Check sheet for the modelled part. Datum: model origin and axes. Units: mm. Face numbers are marked on the shaded views. A direction names the side the tool comes from. Coordinates: 2 decimals unless noted, no trailing zeros. Write each loop counter-clockwise with the first axis right and the second up, starting at its lowest first coordinate (ties: lowest second). Pieces come first, ordered by that corner, then holes. Notation, with made-up numbers: (76, 49) - (109, 49) arc R15 cw to (109, 55) - close; hole circle Ø4 at (65.5, -35.75). An arc over 180 degrees is marked (long way). Write each question's results on one line, items separated by ' | '.
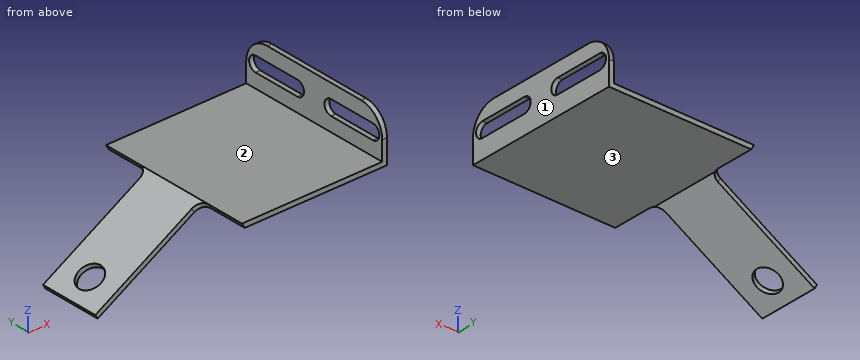
Autodesk Inventor part; units mm, degrees
ref_plane "YZ Plane" through (0, 0, 0) normal (1, 0, 0) x (0, 1, 0)
ref_plane "XZ Plane" through (0, 0, 0) normal (0, 1, 0) x (-1, 0, 0)
ref_plane "XY Plane" through (0, 0, 0) normal (0, 0, 1) x (1, 0, 0)
sketch "Skizze1" plane through (0, 0, 0) normal (0, 1, 0) x (-1, 0, 0)
  line L0 (0, 0) -> (0, -2)
  line L1 (0, -2) -> (60, -2)
  line L2 (60, -2) -> (103.3013, -27)
  line L3 (103.3013, -27) -> (104.3013, -25.2679)
  line L4 (0, 0) -> (60.5359, 0)
  line L5 (104.3013, -25.2679) -> (60.5359, 0)
  dimension "d0" = 2
  dimension "d1" = 60
  dimension "d2" = 50
  dimension "d3" = 150
  dimension "d4" = 2
  dimension "d42" = 0
extrude "Extrusion1" add sketch "Skizze1" along normal blind 65
sketch "Skizze2" plane through (-60.5359, 0, 0) normal (0, 0, 1) x (1, 0, 0)
  line L0 (60.5359, 0) -> (0.5359, 0)
  line L1 (60.5359, 0) -> (58.5359, 0)
  line L2 (58.5359, 0) -> (58.5359, 65)
  line L3 (58.5359, 65) -> (60.5359, 65)
  line L4 (60.5359, 65) -> (60.5359, 0)
  point P0 (58.5359, 0)
  dimension "d8" = 2
  dimension "d9" = 65
extrude "Extrusion2" add sketch "Skizze2" along normal blind 18
sketch "Skizze3" plane through (-2, 0, 0) normal (-1, 0, 0) x (0, 0, 1)
  line L0 (0, 0) -> (18, 0)
  line L1 (18, 65) -> (18, 0)
  line L2 (9, 24.5) -> (9, 4.5) construction
  line L3 (5.9, 24.5) -> (5.9, 4.5)
  line L4 (12.1, 4.5) -> (12.1, 24.5)
  arc A0 (12.1, 24.5) -> (5.9, 24.5) centre (9, 24.5) ccw
  arc A1 (5.9, 4.5) -> (12.1, 4.5) centre (9, 4.5) ccw
  line L5 (9, 60.5) -> (9, 40.5) construction
  line L6 (5.9, 60.5) -> (5.9, 40.5)
  line L7 (12.1, 40.5) -> (12.1, 60.5)
  arc A2 (12.1, 60.5) -> (5.9, 60.5) centre (9, 60.5) ccw
  arc A3 (5.9, 40.5) -> (12.1, 40.5) centre (9, 40.5) ccw
  line L8 (0, 0) -> (0, 65)
  point P0 (9, 14.5)
  point P1 (9, 50.5)
  dimension "d12" = 36
  dimension "d32" = 6.2
  dimension "d34" = 20
  dimension "d35" = 14.5
  dimension "d36" = 6.2
  dimension "d37" = 20
  dimension "d43" = 9
  dimension "d44" = 18
sketch "Skizze4" plane through (-60.5359, 0, 0) normal (-0.5, 0, 0.8660254) x (0.8660254, 0, 0.5)
  line L0 (-50.5359, 0) -> (0, 0)
  line L1 (-50.5359, 0) -> (-50.5359, 65)
  point P0 (52.4256, 0)
  point P1 (-40.5359, 32.5)
  dimension "d23" = 32.5
  dimension "d24" = 10
hole "Bohrung2" at (-95.641, 32.5, -20.2679) direction (0.5, 0, -0.8660254) diameter 10.4 end through all
extrude "Extrusion3" cut sketch "Skizze3" against normal blind 10
fillet "Rundung1" radius 10 4 edges at (-103.8013, 65, -26.134) (-103.8013, 0, -26.134) (-1, 0, 18) (-1, 65, 18)
sketch "Skizze6" plane through (-60.5359, 0, 0) normal (-0.5, 0, 0.8660254) x (0.8660254, 0, 0.5)
  line L0 (0, 0) -> (0, 65)
  line L1 (0, 0) -> (-50.536, 0)
  line L2 (-50.536, 0) -> (-50.536, 20)
  line L3 (-50.536, 20) -> (0, 20)
  line L4 (0, 20) -> (0, 0)
  line L5 (-40.5359, 65) -> (0, 65)
  line L6 (0, 65) -> (-50.536, 65)
  line L7 (-50.536, 65) -> (-50.536, 45)
  line L8 (-50.536, 45) -> (0, 45)
  line L9 (0, 45) -> (0, 65)
  point P0 (52.4256, 0)
  point P1 (0, 45)
  point P2 (0, 20)
  dimension "d46" = 50.536
  dimension "d47" = 20
  dimension "d48" = 50.536
  dimension "d49" = 20
extrude "Extrusion4" cut sketch "Skizze6" against normal blind 10
fillet "Rundung2" radius 4 2 edges at (-59.9585, 20, -1) (-59.9585, 45, -1)
equation "\"d36\" = d32"
equation "\"d37\" = d34"
equation "\"d43\" = 0.5 * d44"
properties part number "Lampenhalterung 2,0"
1. Sectioned sample at B-B (y = 29). Record the cut outline in (x, z) (3 decimals).
Values follow:
outline: (-104.301, -25.268) - (-103.301, -27) - (-97.972, -23.923) - (-98.972, -22.191) - close; (-92.31, -18.345) - (-91.31, -20.077) - (-60, -2) - (0, -2) - (0, 18) - (-2, 18) - (-2, 0) - (-60.536, 0) - close
2. Sectioned sample at D-D (z = -6.5). Record the cut outline in (x, y).
Values follow:
outline: (-71.79, 20) - (-67.79, 20) - (-67.79, 45) - (-71.79, 45) - close
3. Go/stop test with flat-tipped pins: pin 1 (6 mm diameter, centred on y = 35, z = -14.5, fed in from +X); pin 2 (20 mm diameter, centred on x = -91, z = -20, fed in from +Y); pin 3 (7.5 mm diameter, centred on x = -83.5, z = -18.5, fed in from -Y); pin 4 (4 mm diameter, centred on x = -46, z = 2.5, fed in from -Y). Record where each tip stops, or that it passes through.
Values follow:
pin 1: stops at x = -76.45 | pin 2: stops at y = 45 | pin 3: stops at y = 20 | pin 4: passes through
4. Access from +Z, -Z, +X, -X, +Y, -Y to the whole of each face (thin tool, end or side, straight path). Record for the marked faces 1, 2 and 3.
Values follow:
face 1: +Z, -Z, +X, +Y, -Y | face 2: +Z, -X, +Y, -Y | face 3: -Z, +X, +Y, -Y
5. Material ranges on L1, parallel to Z at x = -30, y = 36.5; L2, parallel to X at y = 14.5, z = -0.5, recorded low to high. Write a range as [from, to].
Values follow:
L1: z = [-2, 0] | L2: x = [-60.25, 0]
6. Sectioned sample at A-A (y = 50.5). Record the cut outline in (x, z), then the cut area to 3 significant figures.
Values follow:
outline: (-60.54, 0) - (-59.38, -2) - (0, -2) - (0, 5.9) - (-2, 5.9) - (-2, 0) - close; (-2, 12.1) - (0, 12.1) - (0, 18) - (-2, 18) - close | area: 144 mm^2
7. Sectioned sample at C-C (x = -36). Record the cut outline in (y, z), then the cut area to 3 significant figures.
Values follow:
outline: (0, -2) - (65, -2) - (65, 0) - (0, 0) - close | area: 130 mm^2
